Build history of the part. All positions in model axes, mm. A direction names the side the tool comes from. Round coordinates to 2 decimals unless told otherwise and drop trailing zeros. Loops run counter-clockwise (first coordinate to the right, second up) from the corner with the lowest first, then second, coordinate; pieces in that order, holes last.
from build123d import *

# Parameters (mm, degrees)
F0_W     = 63
F0_H     = 71
F0_W_2   = 60
F0_H_2   = 68
F0_R     = 1.5
F1_DEPTH = 2
F2_DEPTH = 28


with BuildPart() as f1:
    # F0 (on Top) → F1 (new body)
    with BuildSketch(Plane.XY):
        Rectangle(F0_W, F0_H)
        Rectangle(F0_W_2, F0_H_2, mode=Mode.SUBTRACT)
        Rectangle(F0_W_2, F0_H_2)
        Circle(F0_R, mode=Mode.SUBTRACT)
    extrude(amount=F1_DEPTH)

    # F0 (on Top) → F2 (join)
    with BuildSketch(Plane.XY):
        Rectangle(F0_W, F0_H)
        Rectangle(F0_W_2, F0_H_2, mode=Mode.SUBTRACT)
    extrude(amount=F2_DEPTH)


solid = f1.part
(1) Pin check, flat tips, straight feed: P1, Ø18, axis at x = -10, y = -11, coming from the +Z side; P2, Ø4, axis at x = -10, y = -25, coming from the -Z side. Stop position of each tip, or through.
Responses:
P1: stops at z = 2
P2: stops at z = 0
(2) Pull direction X, two halves, no side cores. Call faces 1 (the face through (-31.5, 0, 14)), 2 (the face through (-1.5, 0.07, 0.99)), 3 (the face through (31.5, 0, 14)), 4 (the face through (-30.5, 0.2, 28)): +X half, -X half, draft (parallel to the pull), parting line (faces both ways), or undercut.
Responses:
face 1: -X half
face 2: undercut
face 3: +X half
face 4: draft
(3) Slice it at A-A on x = 0. List the corners of the cut face in (y, z), plus the area to 3 significant figures.
Responses:
outline: (-35.5, 0) - (-1.5, 0) - (-1.5, 2) - (-34, 2) - (-34, 28) - (-35.5, 28) - close; (1.5, 0) - (35.5, 0) - (35.5, 28) - (34, 28) - (34, 2) - (1.5, 2) - close
area: 214 mm2
(4) Slice it at C-C on z = 6.75. List the corners of the cut face in (x, y).
Responses:
outline: (-31.5, -35.5) - (31.5, -35.5) - (31.5, 35.5) - (-31.5, 35.5) - close; hole (-30, -34) - (30, -34) - (30, 34) - (-30, 34) - close
(5) Probe line 1 (X direction, y = -14.5, z = 26.5); line 2 (Y direction, x = -9.5, z = 12.75); line 3 (Y direction, x = 0, z = 1). List the from-to ranges inside material, lowest first.
Responses:
line 1: x = -31.5 to -30, 30 to 31.5
line 2: y = -35.5 to -34, 34 to 35.5
line 3: y = -35.5 to -1.5, 1.5 to 35.5
(6) Which spindle directions (+Z, -Z, +X, -X, +Y, -Y) get a long thin tool onto all of the face, cutting with end or side? Do faces 5 (the face through (0, -35.5, 14)), 6 (the face through (-30, 0, 15)). Say none if no direction does.
Responses:
face 5: +Z, -Z, +X, -X, -Y
face 6: +Z
(7) Slice it at D-D on y = -22.5. List the corners of the cut face in (x, z), plus the area to 3 significant figures.
Responses:
outline: (-31.5, 0) - (31.5, 0) - (31.5, 28) - (30, 28) - (30, 2) - (-30, 2) - (-30, 28) - (-31.5, 28) - close
area: 204 mm2
(8) Slice it at B-B on y = 0. List the corners of the cut face in (x, z), plus the area to 3 significant figures.
Responses:
outline: (-31.5, 0) - (-1.5, 0) - (-1.5, 2) - (-30, 2) - (-30, 28) - (-31.5, 28) - close; (1.5, 0) - (31.5, 0) - (31.5, 28) - (30, 28) - (30, 2) - (1.5, 2) - close
area: 198 mm2
